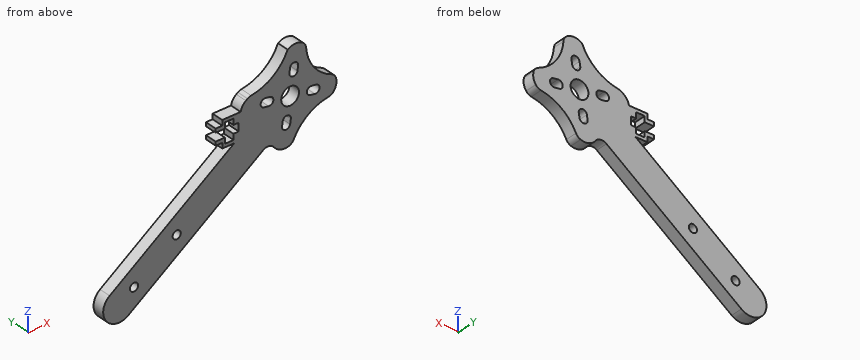
```python
from build123d import *

# Parameters (mm, degrees)
SKETCH_3_R          = 3.375
SKETCH_3_R_2        = 1.55
EXTRUDE_1_DEPTH     = 4.5
FILLET_1_R          = 5
CUT_EXTRUDE_2_REACH = 154.257
FILLET_3_R          = 3


# Some blends are built 0.0001 mm under size
with BuildPart() as part:
    # 草图3 → 凸台-拉伸1 (new body)
    with BuildSketch(Plane(origin=(0, 0, 0), x_dir=(1, 0, 0), z_dir=(0, 1, 0))):
        with BuildLine():
            Line((41.866639538, -23.001486264), (95.429117628, -61.916904502))
            Line((95.429117628, -61.916904502), (100.131399646, -55.444768547))
            Line((100.131399646, -55.444768547), (122.783875489, -71.902755611))
            Line((122.783875489, -71.902755611), (106.325888424, -94.555231453))
            Line((106.325888424, -94.555231453), (83.673412582, -78.097244389))
            Line((83.673412582, -78.097244389), (84.470607294, -77))
            Line((84.470607294, -77), (82.009778971, -77))
            Line((82.009778971, -77), (77.5, -77))
            Line((77.5, -77), (77.5, -75))
            Line((77.5, -75), (75, -75))
            Line((75, -75), (75, -73.55))
            Line((75, -73.55), (78.5, -73.55))
            Line((78.5, -73.55), (78.5, -75.75))
            Line((78.5, -75.75), (81.75, -75.75))
            Line((81.75, -75.75), (81.75, -73.55))
            Line((81.75, -73.55), (83.75, -73.55))
            Line((83.75, -73.55), (83.75, -70.45))
            Line((83.75, -70.45), (81.75, -70.45))
            Line((81.75, -70.45), (81.75, -68.25))
            Line((81.75, -68.25), (78.5, -68.25))
            Line((78.5, -68.25), (78.5, -70.45))
            Line((78.5, -70.45), (75, -70.45))
            Line((75, -70.45), (75, -69))
            Line((75, -69), (77.5, -69))
            Line((77.5, -69), (77.5, -67))
            Line((77.5, -67), (82.009778971, -67))
            Line((82.009778971, -67), (34.81321651, -32.709690196))
            ThreePointArc((34.81321651, -32.709690196), (33.485826058, -24.328876716), (41.866639538, -23.001486264))
        make_face()
        with Locations(Location((103.228644035, -75, 0), (0, 0, 270))):
            Circle(SKETCH_3_R, mode=Mode.SUBTRACT)
        with Locations(Location((44.044221455, -32, 0), (0, 0, 270))):
            Circle(SKETCH_3_R_2, mode=Mode.SUBTRACT)
        with Locations(Location((60.224561343, -43.755705046, 0), (0, 0, 270))):
            Circle(SKETCH_3_R_2, mode=Mode.SUBTRACT)
        with BuildLine():
            Line((110.887677339, -72.217607352), (112.616131935, -71.943847038))
            ThreePointArc((112.616131935, -71.943847038), (114.389522284, -73.232290545), (113.101078777, -75.005680894))
            Line((113.101078777, -75.005680894), (111.372624181, -75.279441208))
            ThreePointArc((111.372624181, -75.279441208), (109.599233832, -73.9909977), (110.887677339, -72.217607352))
        make_face(mode=Mode.SUBTRACT)
        with BuildLine():
            Line((103.508085243, -66.856019854), (103.234324929, -65.127565258))
            ThreePointArc((103.234324929, -65.127565258), (101.46093458, -63.839121751), (100.172491073, -65.6125121))
            Line((100.172491073, -65.6125121), (100.446251387, -67.340966696))
            ThreePointArc((100.446251387, -67.340966696), (102.219641736, -68.629410203), (103.508085243, -66.856019854))
        make_face(mode=Mode.SUBTRACT)
        with BuildLine():
            Line((95.569610731, -77.782392648), (93.841156135, -78.056152962))
            ThreePointArc((93.841156135, -78.056152962), (92.067765787, -76.767709455), (93.356209294, -74.994319106))
            Line((93.356209294, -74.994319106), (95.08466389, -74.720558792))
            ThreePointArc((95.08466389, -74.720558792), (96.858054238, -76.0090023), (95.569610731, -77.782392648))
        make_face(mode=Mode.SUBTRACT)
        with BuildLine():
            Line((102.949202828, -83.143980146), (103.222963142, -84.872434742))
            ThreePointArc((103.222963142, -84.872434742), (104.99635349, -86.160878249), (106.284796997, -84.3874879))
            Line((106.284796997, -84.3874879), (106.011036684, -82.659033304))
            ThreePointArc((106.011036684, -82.659033304), (104.237646335, -81.370589797), (102.949202828, -83.143980146))
        make_face(mode=Mode.SUBTRACT)
    extrude(amount=EXTRUDE_1_DEPTH)

    # 圆角-美观1
    # the kernel refuses this fillet: 5 mm, written as the material it takes off along each edge
    with BuildSketch(Plane(origin=(83.673412582, -8.559797701, 78.097244389), x_dir=(0.5877852522924398, 0, -0.8090169943749717), z_dir=(0, 1, 0))) as fillet_1_piece_1:
        with BuildLine():
            CenterArc((5, -3.423919081), FILLET_1_R, 136.781392116, 43.218607884)
            Line((0, -3.423919081), (-0.1, -3.423919081))
            Line((-0.1, -3.423919081), (-0.1, 0))
            Line((-0.1, 0), (0, 0.1))
            ThreePointArc((0, 0.1), (0.678134326, 0.1), (1.283394026, 0.068478382))
            Line((1.283394026, 0.068478382), (1.356268653, 0))
        make_face()
    extrude(amount=21.619595403, mode=Mode.SUBTRACT)
    with BuildSketch(Plane(origin=(100.131399646, -12.5, 55.444768547), x_dir=(0.8090169943749468, 0, 0.5877852522924739), z_dir=(0, 1, 0)), Plane(origin=(122.783875489, -12.5, 71.902755611), x_dir=(-0.5877852522924745, 0, 0.8090169943749465), z_dir=(0, 1, 0)), Plane(origin=(106.325888424, -12.5, 94.555231453), x_dir=(-0.8090169943749468, 0, -0.5877852522924739), z_dir=(0, 1, 0))) as fillet_1_piece_2:
        with BuildLine():
            CenterArc((FILLET_1_R, -FILLET_1_R), FILLET_1_R, 90, 90)
            Line((0, -FILLET_1_R), (-FILLET_1_R * 0.02, -FILLET_1_R))
            Line((-FILLET_1_R * 0.02, -FILLET_1_R), (-FILLET_1_R * 0.02, FILLET_1_R * 0.02))
            Line((-FILLET_1_R * 0.02, FILLET_1_R * 0.02), (FILLET_1_R, FILLET_1_R * 0.02))
            Line((FILLET_1_R, FILLET_1_R * 0.02), (FILLET_1_R, 0))
        make_face()
    extrude(amount=29.5, mode=Mode.SUBTRACT)

    # 草图4 → 圆弧-美观2 (cut, up to next)
    with BuildSketch(Plane(origin=(0, 4.5, 0), x_dir=(1, 0, 0), z_dir=(0, 1, 0)), mode=Mode.PRIVATE) as cut_extrude_2_sk1:
        with BuildLine():
            Line((104.176484618, -58.383694808), (118.738790517, -68.963829349))
            ThreePointArc((118.738790517, -68.963829349), (109.994899962, -65.687047674), (104.176484618, -58.383694808))
        make_face()
    cut_extrude_2_tool1 = extrude(cut_extrude_2_sk1.sketch, amount=-CUT_EXTRUDE_2_REACH, mode=Mode.PRIVATE) & part.part
    # 草图4 → 圆弧-美观2 (cut, up to next)
    with BuildSketch(Plane(origin=(0, 4.5, 0), x_dir=(1, 0, 0), z_dir=(0, 1, 0)), mode=Mode.PRIVATE) as cut_extrude_2_sk2:
        with BuildLine():
            Line((119.844949227, -75.947840583), (109.264814686, -90.510146481))
            ThreePointArc((109.264814686, -90.510146481), (112.204348353, -81.521230905), (119.844949227, -75.947840583))
        make_face()
    cut_extrude_2_tool2 = extrude(cut_extrude_2_sk2.sketch, amount=-CUT_EXTRUDE_2_REACH, mode=Mode.PRIVATE) & part.part
    # 草图4 → 圆弧-美观2 (cut, up to next)
    with BuildSketch(Plane(origin=(0, 4.5, 0), x_dir=(1, 0, 0), z_dir=(0, 1, 0)), mode=Mode.PRIVATE) as cut_extrude_2_sk3:
        with BuildLine():
            Line((87.718497554, -81.036170651), (102.280803453, -91.616305192))
            ThreePointArc((102.280803453, -91.616305192), (96.462388109, -84.312952326), (87.718497554, -81.036170651))
        make_face()
    cut_extrude_2_tool3 = extrude(cut_extrude_2_sk3.sketch, amount=-CUT_EXTRUDE_2_REACH, mode=Mode.PRIVATE) & part.part
    add(cut_extrude_2_tool1.solids().sort_by_distance((110.868828, 4.5, 64.48419))[0], mode=Mode.SUBTRACT)
    add(cut_extrude_2_tool2.solids().sort_by_distance((113.606622, 4.5, 82.540042))[0], mode=Mode.SUBTRACT)
    add(cut_extrude_2_tool3.solids().sort_by_distance((95.58846, 4.5, 85.51581))[0], mode=Mode.SUBTRACT)

    # 圆角-美观3
    fillet_3_edges = [part.edges().sort_by_distance(p)[0] for p in [
        (104.176484618, 2.25, 58.383694808),
        (118.738790517, 2.25, 68.963829349),
        (119.844949227, 2.25, 75.947840583),
        (109.264814686, 2.25, 90.510146481),
        (95.429117628, 2.25, 61.916904502),
        (87.718497554, 2.25, 81.036170651),
    ]]
    fillet(fillet_3_edges, radius=FILLET_3_R - 0.0001)  # a hair under: the kernel refuses the full size


solid = part.part
```
Design review of the part built by this model. Coordinates are the model's own, in mm. Coordinates: 2 decimals unless noted, no trailing zeros. Write each loop counter-clockwise with the first axis right and the second up, starting at its lowest first coordinate (ties: lowest second). Pieces come first, ordered by that corner, then holes.
1) Add section A-A (y = 2.55). State how many separate pieces and enclosed holes the cut face has, plus the area to 3 significant figures.
2) To check wall thickness, follow L1, parallel to Z at x = 76, y = 0.95; L2, parallel to X at y = 1.3, z = 32; L3, parallel to X at y = 2.1, z = 64.5. State the ranges of each line that lie inside material, in increasing order.
3) Add section C-C (z = 39.5). Write out the cut boundary in (x, y).
4) Insertion check: pin 1 (0.6 mm diameter, centred on y = 3, z = 68.5, fed in from -X); pin 2 (0.8 mm diameter, centred on x = 77, y = 2, fed in from -Z); pin 3 (2 mm diameter, centred on x = 83, y = 1.5, fed in from +Z). Each pin has a flat end and moves straight along its axis. Give the tip position at first contact, or say it passes through.
5) Add section B-B (x = 72.5). Write out the cut boundary in (y, z), plus the area to 3 significant figures.
Check result:
1. separate pieces: 1
1. enclosed holes: 7
1. area: 1,480 mm2
2. L1: z = 47.8 to 62.63, 69 to 70.45, 73.55 to 75
2. L2: x = 34 to 42.49, 45.59 to 54.25
2. L3: x = 78.57 to 100.42, 102.99 to 108.53
3. outline: (44.16, 0) - (64.57, 0) - (64.57, 4.5) - (44.16, 4.5) - close
4. pin 1: stops at x = 77.5
4. pin 2: stops at z = 48.24
4. pin 3: stops at z = 77
5. outline: (0, 45.26) - (4.5, 45.26) - (4.5, 60.09) - (0, 60.09) - close
5. area: 66.7 mm2
